The listing builds one solid part. Answer for the finished solid, in the listing's coordinates (mm). A direction names the side the tool comes from. Give positions to 0.01 mm unless a question says otherwise; leave off trailing zeros. Write each loop counter-clockwise with the first axis right and the second up, starting at its lowest first coordinate (ties: lowest second). Pieces come first, ordered by that corner, then holes. Notation, with made-up numbers: (-25, 41) - (-3, 41) arc R24 cw to (-3, 57) - close; hole circle Ø8 at (27, 14). An arc over 180 degrees is marked (long way). One line per question, with ' | ' between items. Start each with the question number.
1. For faces 1 (the face through (-17, 3, 16)), 2 (the face through (-67.97, 2.55, 17.32)), 3 (the face through (0, 17, 17)), 4 (the face through (-34, 17, 34.2)), 5 (the face through (-50.589, 31.836, 15.636)), determine the directions among +Z, -Z, +X, -X, +Y, -Y from which every point of the face is accessible in a straight line to the end or side of a thin tool.
2. The mould has two halves that part along Y. Classify faces 6 (the face through (-67.95, 33.77, 17.32)), 7 (the face through (-52, 17, 3)), 8 (the face through (-0.43, 17.32, 0.45)): +Y half, -Y half, draft (parallel to the pull), parting line (faces both ways), or undercut.
3. Find the intervals of material crossed by L1, parallel to Z at x = -59, y = 11; L2, parallel to Z at x = -34.6, y = 17.1, in increasing order. Write a range as from..to.
4. Given P1, Ø14, axis at y = 17.5, z = 14.5, coming from the -X side; P2, Ø14, axis at x = -21, y = 19, coming from the -Z side; P3, Ø4, axis at x = -17.05, z = 17.1, coming from the +Y side, each flat-ended and moving along its own axis, determine where each tip first touches the part or whether it passes through.
5. A cutting plane is placed at D-D (x = -45). Determine the outline of the cut face in (y, z).
```python
from build123d import *

# Parameters (mm, degrees)
F1_DEPTH             = 34.2
F2_W                 = 34.2
F2_H                 = 34.2
F3_DEPTH             = 34.2
F4_W                 = 28.2
F4_H                 = 28.2
F5_DEPTH             = 31.2
F8_D                 = 3.3
F8_DEPTH             = 25
F8_CSINK_D           = 6.72
F8_CSINK_ANGLE       = 90
F8_TIP               = 0.9914200214
F8_ON_F7_D           = 3.3
F8_ON_F7_DEPTH       = 25
F8_ON_F7_CSINK_D     = 6.72
F8_ON_F7_CSINK_ANGLE = 90
F8_ON_F7_TIP         = 0.9914200214
F9_W                 = 28.2
F9_H                 = 28.2
F10_DEPTH            = 31.2
F11_R                = 1.49999
F12_W                = 5
F12_H                = 5
F13_DEPTH            = 2.5


# Not quite as in the source:
# - a fillet or chamfer is up to 0.001 mm smaller than in the source, because OpenCascade refuses the exact size
# - a feature names something its author has since deleted; it is built from what else it names


with BuildPart() as f1:
    # F0 (on Top) → F1 (new body)
    with BuildSketch(Plane.XY):
        Polygon((-34.2, 0), (-8, 0), (0, 0), (0, 34.2), (-34.2, 34.2), align=None)
    extrude(amount=F1_DEPTH)

    # F2 (on face) → F3 (join)
    with BuildSketch(Plane(origin=(-34.2, 0, 0), x_dir=(0, -1, 0), z_dir=(-1, 0, 0))):
        with Locations((-17.1, 17.1)):
            Rectangle(F2_W, F2_H)
    extrude(amount=F3_DEPTH)

    # F4 (on face) → F5 (cut)
    with BuildSketch(Plane(origin=(-68.4, 0, 0), x_dir=(0, -1, 0), z_dir=(-1, 0, 0))):
        with Locations((-17.1, 17.1)):
            Rectangle(F4_W, F4_H)
    extrude(amount=-F5_DEPTH, mode=Mode.SUBTRACT)

    # F8
    with Locations(Plane(origin=(0, 34.2, 0), x_dir=(-1, 0, 0), z_dir=(0, 1, 0))):
        with Locations((17.05, 17.1), (51.35, 17.1)):
            CounterSinkHole(F8_D / 2, F8_CSINK_D / 2, depth=F8_DEPTH, counter_sink_angle=F8_CSINK_ANGLE)
            with Locations((0, 0, -(F8_DEPTH + F8_TIP / 2))):  # 118° drill point
                Cone(0, F8_D / 2, F8_TIP, mode=Mode.SUBTRACT)

    # F8 on F7
    with Locations(Plane(origin=(-37.2, 0, 0), x_dir=(0, -1, 0), z_dir=(-1, 0, 0))):
        with Locations((-17.1, 17.1)):
            CounterSinkHole(F8_ON_F7_D / 2, F8_ON_F7_CSINK_D / 2, depth=F8_ON_F7_DEPTH, counter_sink_angle=F8_ON_F7_CSINK_ANGLE)
            with Locations((0, 0, -(F8_ON_F7_DEPTH + F8_ON_F7_TIP / 2))):  # 118° drill point
                Cone(0, F8_ON_F7_D / 2, F8_ON_F7_TIP, mode=Mode.SUBTRACT)

    # F9 (on face) → F10 (cut)
    with BuildSketch(Plane(origin=(0, 0, 0), x_dir=(1, 0, 0), z_dir=(0, 0, -1))):
        with Locations((-17.1, -17.1)):
            Rectangle(F9_W, F9_H)
    extrude(amount=-F10_DEPTH, mode=Mode.SUBTRACT)

    # F11 (radius 1.5 in the source; OpenCascade refuses exactly that, so slightly less here)
    f11_edges = [f1.edges().sort_by_distance(p)[0] for p in [
        (-31.2, 17.1, 0),
        (-17.1, 3, 0),
        (-3, 17.1, 0),
        (-17.1, 31.2, 0),
        (-34.2, 34.2, 0),
        (-34.2, 0, 0),
        (0, 17.1, 0),
        (-68.4, 17.1, 0),
        (-68.4, 0, 17.1),
        (-68.4, 17.1, 34.2),
        (-68.4, 34.2, 17.1),
        (-68.4, 17.1, 31.2),
        (-68.4, 3, 17.1),
        (-68.4, 17.1, 3),
        (-68.4, 31.2, 17.1),
        (-34.2, 0, 34.2),
        (-34.2, 34.2, 34.2),
        (0, 17.1, 34.2),
        (0, 34.2, 17.1),
        (0, 0, 17.1),
    ]]
    fillet(f11_edges, radius=F11_R)

    # F12 (on face) → F13 (cut)
    with BuildSketch(Plane(origin=(0, 34.2, 0), x_dir=(-1, 0, 0), z_dir=(0, 1, 0))):
        with Locations((14.5, 25.7)):
            Rectangle(F12_W, F12_H)
    extrude(amount=-F13_DEPTH, mode=Mode.SUBTRACT)


solid = f1.part
```
Determined:
1) face 1: -Z | face 2: -X | face 3: +Z, -Z, +X, +Y, -Y | face 4: +Z, +X, -X, +Y, -Y | face 5: +Y
2) face 6: +Y half | face 7: undercut | face 8: draft
3) L1: 0..3, 31.2..34.2 | L2: 0..15.45, 18.75..34.2
4) P1: x = -37.2 | P2: z = 31.2 | P3: y = 32.84
5) outline: (0, 1.5) arc R1.5 ccw to (1.5, 0) - (32.7, 0) arc R1.5 ccw to (34.2, 1.5) - (34.2, 32.7) arc R1.5 ccw to (32.7, 34.2) - (1.5, 34.2) arc R1.5 ccw to (0, 32.7) - close; hole (3, 3) - (31.2, 3) - (31.2, 31.2) - (3, 31.2) - close
